Autodesk Inventor part; units mm, degrees
ref_plane "YZ Plane" through (0, 0, 0) normal (1, 0, 0) x (0, 1, 0)
ref_plane "XZ Plane" through (0, 0, 0) normal (0, 1, 0) x (-1, 0, 0)
ref_plane "XY Plane" through (0, 0, 0) normal (0, 0, 1) x (1, 0, 0)
sketch "Esquisse2" plane through (0, 0, 0) normal (0, 0, 1) x (1, 0, 0)
  line L0 (-26, -17.5) -> (26, -17.5)
  line L1 (26, -17.5) -> (26, 17.5)
  line L2 (26, 17.5) -> (-26, 17.5)
  line L3 (-26, 17.5) -> (-26, -17.5)
  line L4 (-26, -17.5) -> (26, 17.5) construction
  line L5 (26, -17.5) -> (-26, 17.5) construction
  point P0 (0, 0)
  dimension "d0" = 52
  dimension "d1" = 35
extrude "Extrusion1" add sketch "Esquisse2" along normal blind 5
sketch "Esquisse3" plane through (26, -17.5, 0) normal (1, 0, 0) x (0, 0, -1)
  line L0 (0, 0) -> (0, 35) construction
  line L1 (0, 35) -> (-5, 35) construction
  line L2 (-5, 0) -> (-5, 35) construction
  line L3 (0, 0) -> (-5, 0) construction
  line L4 (0, 17.5) -> (-2.5, 17.5) construction
  line L5 (-1.75, 0) -> (-3.25, 0)
  line L6 (-3.25, 0) -> (-3.25, 35)
  line L7 (-3.25, 35) -> (-1.75, 35)
  line L8 (-1.75, 35) -> (-1.75, 0)
  line L9 (-1.75, 0) -> (-3.25, 35) construction
  line L10 (-3.25, 0) -> (-1.75, 35) construction
  dimension "d4" = 2.5
  dimension "d5" = 1.5
extrude "Extrusion2" add sketch "Esquisse3" along normal blind 1.5
mirror "Symétrie1" about plane through (0, 0, 0) normal (1, 0, 0) of "Extrusion2"
sketch "Esquisse4" plane through (0, 0, 5) normal (0, 0, 1) x (1, 0, 0)
  line L0 (-26, 17.5) -> (-26, -17.5) construction
  line L1 (-26, -17.5) -> (26, -17.5) construction
  line L2 (26, -17.5) -> (26, 17.5) construction
  line L3 (26, 17.5) -> (-26, 17.5) construction
  line L4 (-26, -17.5) -> (26, -17.5)
  line L5 (26, -17.5) -> (26, -15)
  line L6 (26, -15) -> (-26, -15)
  line L7 (-26, -15) -> (-26, -17.5)
  point P0 (0, 0)
  dimension "d8" = 2.5
extrude "Extrusion3" add sketch "Esquisse4" along normal blind 5
sketch "Esquisse5" plane through (-26, 17.5, 0) normal (0, 1, 0) x (1, 0, 0)
  line L0 (52, 0) -> (0, 0) construction
  line L1 (0, 0) -> (0, -1.75) construction
  line L2 (0, -1.75) -> (-1.5, -1.75) construction
  line L3 (-1.5, -1.75) -> (-1.5, -3.25) construction
  line L4 (0, -3.25) -> (-1.5, -3.25) construction
  line L5 (0, -3.25) -> (0, -5) construction
  line L6 (52, -5) -> (0, -5) construction
  line L7 (52, -3.25) -> (52, -5) construction
  line L8 (52, -3.25) -> (53.5, -3.25) construction
  line L9 (53.5, -1.75) -> (53.5, -3.25) construction
  line L10 (52, -1.75) -> (53.5, -1.75) construction
  line L11 (52, 0) -> (52, -1.75) construction
  line L12 (26, 2) -> (26, -12) construction
  line L13 (-12.5, 0) -> (64.5, 0) construction
  line L14 (26, 0) -> (30, 0) construction
  line L15 (30, 0) -> (22, 0)
  line L16 (22, 0) -> (22, -3)
  line L17 (22, -3) -> (30, -3)
  line L18 (30, -3) -> (30, 0)
  dimension "d11" = 4
  dimension "d12" = 8
  dimension "d13" = 3
extrude "Extrusion4" add sketch "Esquisse5" along normal blind 8.5
fillet "Congé1" radius 2 2 edges at (4, 26, 1.5) (-4, 26, 1.5)
fillet "Congé1" radius 4 2 edges at (0, -17.5, 0) (0, -15, 5)
sketch "Esquisse6" plane through (-4, 17.5, 3) normal (0, 0, 1) x (1, 0, 0)
  line L0 (30, -28.5) -> (-22, -28.5) construction
  line L1 (30, -28.5) -> (30, 0) construction
  line L2 (30, 0) -> (-22, 0) construction
  line L3 (-22, 0) -> (-22, -28.5) construction
  arc A0 (2, 8.5) -> (0, 6.5) centre (2, 6.5) ccw construction
  line L4 (0, 0) -> (0, 6.5) construction
  line L5 (8, 0) -> (0, 0) construction
  line L6 (8, 0) -> (8, 6.5) construction
  arc A1 (8, 6.5) -> (6, 8.5) centre (6, 6.5) ccw construction
  line L7 (2, 8.5) -> (6, 8.5) construction
  line L8 (4, 0) -> (4, 4.5) construction
  circle A2 centre (4, 4.5) radius 1.75
  point P0 (4, -17.5)
  dimension "d18" = 4.5
  dimension "d19" = 3.5
extrude "Extrusion5" cut sketch "Esquisse6" against normal through all
properties part number "_Impression 3D"
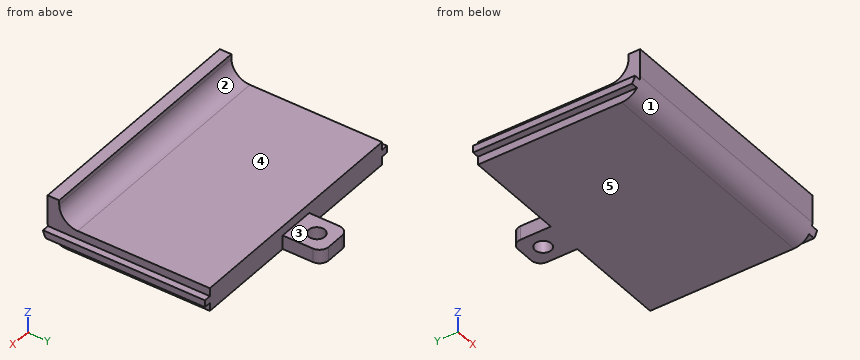
Design review of the part built by this model. Coordinates are the model's own, in mm. Face numbers are marked on the shaded views. A direction names the side the tool comes from. Give positions to 0.01 mm unless a question says otherwise; leave off trailing zeros. Order: outer loops, then holes, each group sorted by start corner. A loop starts at its lowest first (then second) coordinate and runs counter-clockwise, first axis right, second up. Notation, with made-up numbers: (-6, 42.25) - (47, 42.25) arc R36 ccw to (47, 80.25) - close; hole circle Ø8 at (-7.5, 19). An arc over 180 degrees is marked (long way). Use a Markdown table: item, result. Add a question column.
(1) Add section A-A on y = 22. Give the boundary of the cut face in (x, z).
(2) Wall thickness on probe 1 along Z at (x, y) = (6, -2.5); probe 2 along X at (y, z) = (-4.5, 4); probe 3 along Y at (x, z) = (-5.5, 3.25): over which ranges is each line inside the solid? List them lowest first. Write a range as [from, to].
(3) Mouldability with a two-part tool opening along Y and no side actions: class the marked faces 1, 2 and 3 as +Y half, -Y half, draft (parallel to the pull), parting line (faces both ways), or undercut.
(4) Add section B-B on x = 0. Give the boundary of the cut face in (y, z), then the cut area to 4 significant figures.
(5) Machinability: for the marked faces 4 and 5, which of the approach directions +Z, -Z, +X, -X, +Y, -Y give a long, thin tool a straight path to every point of the face, cutting with its end or side? Answer none if there is none.
(6) Add section D-D on z = 6.25. Give the boundary of the cut face in (x, y).
(7) Clearance check with flat-ended pins moving along their axes: P1, Ø2, axis at x = -5, z = 7.5, coming from the +Y side; P2, Ø1.5, axis at x = -6, z = 3, coming from the +Y side; P3, Ø0.9, axis at y = -1.5, z = 0.5, coming from the +X side. State where each tip first meets the part, or that it passes through.
(8) Add section C-C on y = -9. Give the boundary of the cut face in (x, z), then the cut area to 4 significant figures.
Report:
| question | item | result |
|---|---|---|
| 1 | outline | (-4, 0) - (-1.75, 0) - (-1.75, 3) - (-4, 3) - close; (1.75, 0) - (4, 0) - (4, 3) - (1.75, 3) - close |
| 2 | probe 1 | z = [0, 5] |
| 2 | probe 2 | x = [-26, 26] |
| 2 | probe 3 | y = [-17.43, 17.5] |
| 3 | face 1 | -Y half |
| 3 | face 2 | +Y half |
| 3 | face 3 | draft |
| 4 | outline | (-17.5, 4) arc R4 ccw to (-13.5, 0) - (20.25, 0) - (20.25, 3) - (17.5, 3) - (17.5, 5) - (-11, 5) arc R4 cw to (-15, 9) - (-15, 10) - (-17.5, 10) - close; (23.75, 0) - (26, 0) - (26, 3) - (23.75, 3) - close |
| 4 | area | 202.5 mm² |
| 5 | face 4 | +Z, +X, -X, +Y |
| 5 | face 5 | -Z, +X, -X, +Y, -Y |
| 6 | outline | (-26, -17.5) - (26, -17.5) - (26, -13.9) - (-26, -13.9) - close |
| 7 | P1 | stops at y = -14.12 |
| 7 | P2 | stops at y = 17.5 |
| 7 | P3 | stops at x = 26 |
| 8 | outline | (-27.5, 1.75) - (-26, 1.75) - (-26, 0) - (26, 0) - (26, 1.75) - (27.5, 1.75) - (27.5, 3.25) - (26, 3.25) - (26, 5) - (-26, 5) - (-26, 3.25) - (-27.5, 3.25) - close |
| 8 | area | 264.5 mm² |
